```python
from build123d import *

# Parameters (mm, degrees)
BOSS_EXTRUDE1_DEPTH = 55
SKETCH2_R           = 9.5
CUT_EXTRUDE1_DEPTH  = 60
SKETCH3_R           = 19.5
CUT_EXTRUDE2_DEPTH  = 3
SKETCH4_R           = 2.5
CUT_EXTRUDE3_DEPTH  = 23
SKETCH5_W           = 5
SKETCH5_H           = 5
CUT_EXTRUDE4_DEPTH  = 5
CUT_EXTRUDE5_DEPTH  = 60
SKETCH7_R           = 1.5
BOSS_EXTRUDE2_DEPTH = 5


with BuildPart() as part:
    # Sketch1 → Boss-Extrude1 (new body)
    with BuildSketch(Plane(origin=(0, 0, 0), x_dir=(1, 0, 0), z_dir=(0, 1, 0))):
        Polygon((-28.867513459, 0), (-14.43375673, -25), (14.43375673, -25), (28.867513459, 0), (14.43375673, 25), (-14.43375673, 25), align=None)
    extrude(amount=BOSS_EXTRUDE1_DEPTH)

    # Sketch2 → Cut-Extrude1 (cut)
    with BuildSketch(Plane.XZ):
        with Locations(Location((0, 0, 0), (0, 0, 270))):
            Circle(SKETCH2_R)
    extrude(amount=-CUT_EXTRUDE1_DEPTH, mode=Mode.SUBTRACT)

    # Sketch3 → Cut-Extrude2 (cut)
    with BuildSketch(Plane(origin=(0, 55, 0), x_dir=(1, 0, 0), z_dir=(0, 1, 0))):
        with Locations(Location((0, 0, 0), (0, 0, 270))):
            Circle(SKETCH3_R)
    extrude(amount=-CUT_EXTRUDE2_DEPTH, mode=Mode.SUBTRACT)

    # Sketch4 → Cut-Extrude3 (cut)
    with BuildSketch(Plane.XY.offset(25)):
        with Locations((0, 12)):
            Circle(SKETCH4_R)
        with Locations((0, 20)):
            Circle(SKETCH4_R)
        with Locations((0, 28)):
            Circle(SKETCH4_R)
        with Locations((0, 36)):
            Circle(SKETCH4_R)
        with Locations((0, 44)):
            Circle(SKETCH4_R)
    extrude(amount=-CUT_EXTRUDE3_DEPTH, mode=Mode.SUBTRACT)

    # Sketch5 → Cut-Extrude4 (cut)
    with BuildSketch(Plane(origin=(0, 52, 0), x_dir=(1, 0, 0), z_dir=(0, 1, 0))):
        with Locations((-14.134558147, 0)):
            Rectangle(SKETCH5_W, SKETCH5_H)
        with Locations((14.623643585, 0)):
            Rectangle(SKETCH5_W, SKETCH5_H)
    extrude(amount=-CUT_EXTRUDE4_DEPTH, mode=Mode.SUBTRACT)

    # Sketch6 → Cut-Extrude5 (cut)
    with BuildSketch(Plane.XZ):
        Polygon((9.43375673, 25), (-9.43375673, 25), (-11.43375673, 23), (-9.43375673, 23), (9.43375673, 23), (11.43375673, 23), align=None)
    extrude(amount=-CUT_EXTRUDE5_DEPTH, mode=Mode.SUBTRACT)

    # Sketch7 → Boss-Extrude2 (add)
    with BuildSketch(Plane(origin=(0, 55, 0), x_dir=(1, 0, 0), z_dir=(0, 1, 0))):
        with Locations(Location((23.867513459, 0, 0), (0, 0, 270))):
            Circle(SKETCH7_R)
        with Locations(Location((-23.867513459, 0, 0), (0, 0, 270))):
            Circle(SKETCH7_R)
    extrude(amount=BOSS_EXTRUDE2_DEPTH)


solid = part.part
```
Here's how the part is built. I have some questions about the finished solid (model axes, mm). A direction names the side the tool comes from. Give positions to 0.01 mm unless a question says otherwise; leave off trailing zeros. Write each loop counter-clockwise with the first axis right and the second up, starting at its lowest first coordinate (ties: lowest second). Pieces come first, ordered by that corner, then holes. Notation, with made-up numbers: (84.5, 35.5) -> (136.5, 35.5) arc R9 ccw to (136.5, 44.5) -> close; hole circle Ø3 at (38.5, 8.25). An arc over 180 degrees is marked (long way). Write each question's results on one line, items separated by ' | '.
Item 1: Suppose I cut it at B-B on y = 36. Write out the boundary of the cut face in (x, z), plus the area to 3 significant figures.
Output:
outline: (-28.87, 0) -> (-14.43, -25) -> (14.43, -25) -> (28.87, 0) -> (14.43, 25) -> (9.43, 25) -> (11.43, 23) -> (2.5, 23) -> (2.5, 9.17) arc R9.5 cw (long way) to (-2.5, 9.17) -> (-2.5, 23) -> (-11.43, 23) -> (-9.43, 25) -> (-14.43, 25) -> close | area: 1,770 mm^2
Item 2: If I drill on L1, parallel to Y at x = 0, z = 16; L2, parallel to Y at x = 0, z = 20; L3, parallel to X at y = 39.5, z = 0, over which ranges is the centre line in solid material (lowest first)?
Output:
L1: y = 0 to 9.5, 14.5 to 17.5, 22.5 to 25.5, 30.5 to 33.5, 38.5 to 41.5, 46.5 to 52 | L2: y = 0 to 9.5, 14.5 to 17.5, 22.5 to 25.5, 30.5 to 33.5, 38.5 to 41.5, 46.5 to 55 | L3: x = -28.87 to -9.5, 9.5 to 28.87
Item 3: Suppose I cut it at D-D on z = -14. Write out the boundary of the cut face in (x, y).
Output:
outline: (-20.78, 0) -> (20.78, 0) -> (20.78, 55) -> (13.57, 55) -> (13.57, 52) -> (-13.57, 52) -> (-13.57, 55) -> (-20.78, 55) -> close
Item 4: Suppose I cut it at A-A on x = 0. Give the number of separate pieces and of enclosed holes in the cut face, plus the area to 3 significant figures.
Output:
separate pieces: 7 | enclosed holes: 0 | area: 1,200 mm^2
Item 5: For pin 1 Ø7 at (x, y) = (5, 23) entering from +Z; pin 2 Ø1.5 at (x, y) = (-18, 52.5) entering from -Z; pin 3 Ø4 at (y, z) = (49.5, -0.5) entering from +X; pin 4 Ø1 at (x, y) = (20, 23) entering from -Z (3 decimals), each with a flat end and sliding along its axis, tell me the tip position at first contact or that it passes through.
Output:
pin 1: stops at z = 23 | pin 2: stops at z = -20.12 | pin 3: stops at x = 28.87 | pin 4: stops at z = -16.225
Item 6: On a 3-axis mill with a long thin cutter (end or side, diameter ignored), from which of +Z, -Z, +X, -X, +Y, -Y can I reach the whole of each face in a straight line? I mean faces 1 (the face through (-3, 27, 23)), 2 (the face through (17.124, 50, 0)), 3 (the face through (21.55, 27.115, 12.675)). Say none if no direction works.
Output:
face 1: +Y, -Y | face 2: +Y | face 3: +Z, +X, +Y, -Y
Item 7: Suppose I cut it at C-C on x = 7. Write out the boundary of the cut face in (y, z).
Output:
outline: (0, -25) -> (55, -25) -> (55, -18.2) -> (52, -18.2) -> (52, -6.42) -> (0, -6.42) -> close; (0, 6.42) -> (52, 6.42) -> (52, 18.2) -> (55, 18.2) -> (55, 23) -> (0, 23) -> close
Item 8: We'd pull the mould along Z, two halves only. Please class faces 4 (the face through (21.75, 27.12, -12.33)), 5 (the face through (-14, 50, -2.5)), 6 (the face through (-12, 27, 25)): pulls with the +Z half, pulls with the -Z half, needs draft (parallel to the pull), parting line crosses it, or undercut.
Output:
face 4: pulls with the -Z half | face 5: undercut | face 6: pulls with the +Z half
